from build123d import *

# Parameters (mm, degrees)
SKETCH1_R           = 11.049
BOSS_EXTRUDE3_DEPTH = 6.35


with BuildPart() as part:
    # Sketch1 → Boss-Extrude3 (new body)
    with BuildSketch(Plane.XY):
        with BuildLine():
            Line((-15.875, -14.2875), (15.875, -14.2875))
            Line((15.875, -14.2875), (15.875, 1.5875))
            ThreePointArc((15.875, 1.5875), (12.155256121, 10.567756121), (3.175, 14.2875))
            Line((3.175, 14.2875), (-3.175, 14.2875))
            ThreePointArc((-3.175, 14.2875), (-12.155256121, 10.567756121), (-15.875, 1.5875))
            Line((-15.875, 1.5875), (-15.875, -14.2875))
        make_face()
        with Locations((0, -2.8575)):
            Circle(SKETCH1_R, mode=Mode.SUBTRACT)
    extrude(amount=BOSS_EXTRUDE3_DEPTH)


solid = part.part
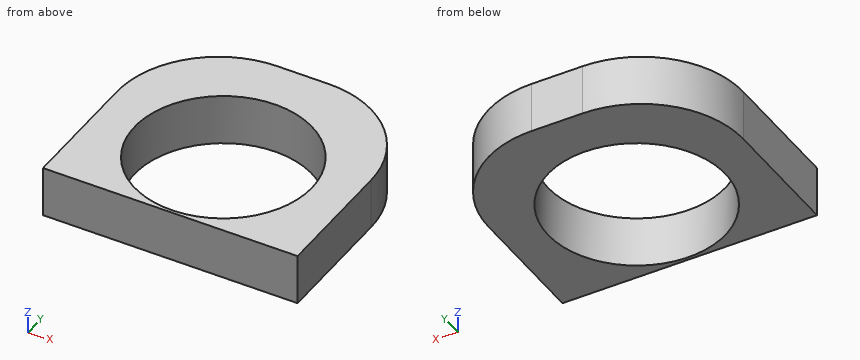
Here's how the part is built. I have some questions about the finished solid (model axes, mm). Give positions to 0.01 mm unless a question says otherwise; leave off trailing zeros. Loops run counter-clockwise (first coordinate to the right, second up) from the corner with the lowest first, then second, coordinate; pieces in that order, holes last. Notation, with made-up numbers: (85, 38.5) -> (97, 38.5) arc R12 ccw to (97, 54.5) -> close; hole circle Ø4 at (79.5, -2). An arc over 180 degrees is marked (long way). Answer as a JSON object with one key per item and string values. Group by question number.
Item 1: Imagine slicing it at A-A on x = 0. Write out the boundary of the cut face in (y, z), then the cut area to 3 significant figures.
Item 2: I need wall thicknesses on L1, parallel to Y at x = 0, z = 3; L2, parallel to X at y = -3, z = 1.25 (3 decimals); L3, parallel to Y at x = 9, z = 2.5. Which ranges of each line are inside material? Lowest first, please.
Item 3: Will these pins go through, and if not, where does the flat tip stop? pin 1 (3 mm diameter, centred on x = -8, y = 0, fed in from -Z); pin 2 (1 mm diameter, centred on x = -12.5, z = 4, fed in from +Y); pin 3 (1 mm diameter, centred on x = 11, z = 4.5, fed in from +Y).
Item 4: Imagine slicing it at B-B on y = 0. Write out the boundary of the cut face in (x, z) (3 decimals), then the cut area to 3 significant figures.
Item 5: Imagine slicing it at D-D on y = 11.5. Write out the boundary of the cut face in (x, z).
Item 6: Imagine slicing it at C-C on z = 2.25. Write out the boundary of the cut face in (x, y) (1 decimal).
Answer list:
{
 "1": {"outline": "(-14.29, 0) -> (-13.91, 0) -> (-13.91, 6.35) -> (-14.29, 6.35) -> close; (8.19, 0) -> (14.29, 0) -> (14.29, 6.35) -> (8.19, 6.35) -> close", "area": "41.1 mm2"},
 "2": {"L1": "y = -14.29 to -13.91, 8.19 to 14.29", "L2": "x = -15.875 to -11.048, 11.048 to 15.875", "L3": "y = -14.29 to -9.27, 3.55 to 12.87"},
 "3": {"pin 1": "passes through", "pin 2": "stops at y = 10.72", "pin 3": "stops at y = 11.96"},
 "4": {"outline": "(-15.875, 0) -> (-10.673, 0) -> (-10.673, 6.35) -> (-15.875, 6.35) -> close; (10.673, 0) -> (15.875, 0) -> (15.875, 6.35) -> (10.673, 6.35) -> close", "area": "66.1 mm2"},
 "5": {"outline": "(-11.11, 0) -> (11.11, 0) -> (11.11, 6.35) -> (-11.11, 6.35) -> close"},
 "6": {"outline": "(-15.9, -14.3) -> (15.9, -14.3) -> (15.9, 1.6) arc R12.7 ccw to (3.2, 14.3) -> (-3.2, 14.3) arc R12.7 ccw to (-15.9, 1.6) -> close; hole circle Ø22.1 at (0, -2.9)"}
}
